Geometry check sheet. Reference: drawing and pictorial views, mm from the part's lowest x, y, z. A direction names the side the tool comes from. Round coordinates to 2 decimals unless told otherwise and drop trailing zeros. Write each loop counter-clockwise with the first axis right and the second up, starting at its lowest first coordinate (ties: lowest second). Pieces come first, ordered by that corner, then holes. Notation, with made-up numbers: M 83,-23.75 L 133,-23.75 A23 cw 133,-8.75 Z; hole C 57.5,89.25 d1. An arc over 180 degrees is marked long. Put each result on its own line as item: value. Start each with the question number.
(1) Tool access check on the marked faces 1, 2 and 3. Record the directions out of +Z, -Z, +X, -X, +Y, -Y that give a thin tool (end or side, any length) a straight path to the whole face; none if there is none.
(2) Section check A-A on z = 38.1. Record the cut outline in (x, y) (3 decimals).
(3) Section check B-B on x = 39. Record the cut outline in (y, z).
(4) Gauge pin test, flat ends, axial feed: pin 1 (6 mm diameter, centred on x = 83, z = 34, fed in from -Y); pin 2 (12 mm diameter, centred on x = 45, z = 63.5, fed in from +Y); pin 3 (12 mm diameter, centred on y = 61, z = 63.5, fed in from +X) (3 decimals). Record the tip position at first contact, or that the pin passes through.
(5) Material ranges on probe 1 along X at (y, z) = (28, 30) (3 decimals); probe 2 along Z at (x, y) = (28.5, 37.5); probe 3 along Y at (x, z) = (55, 60), recorded low to high.
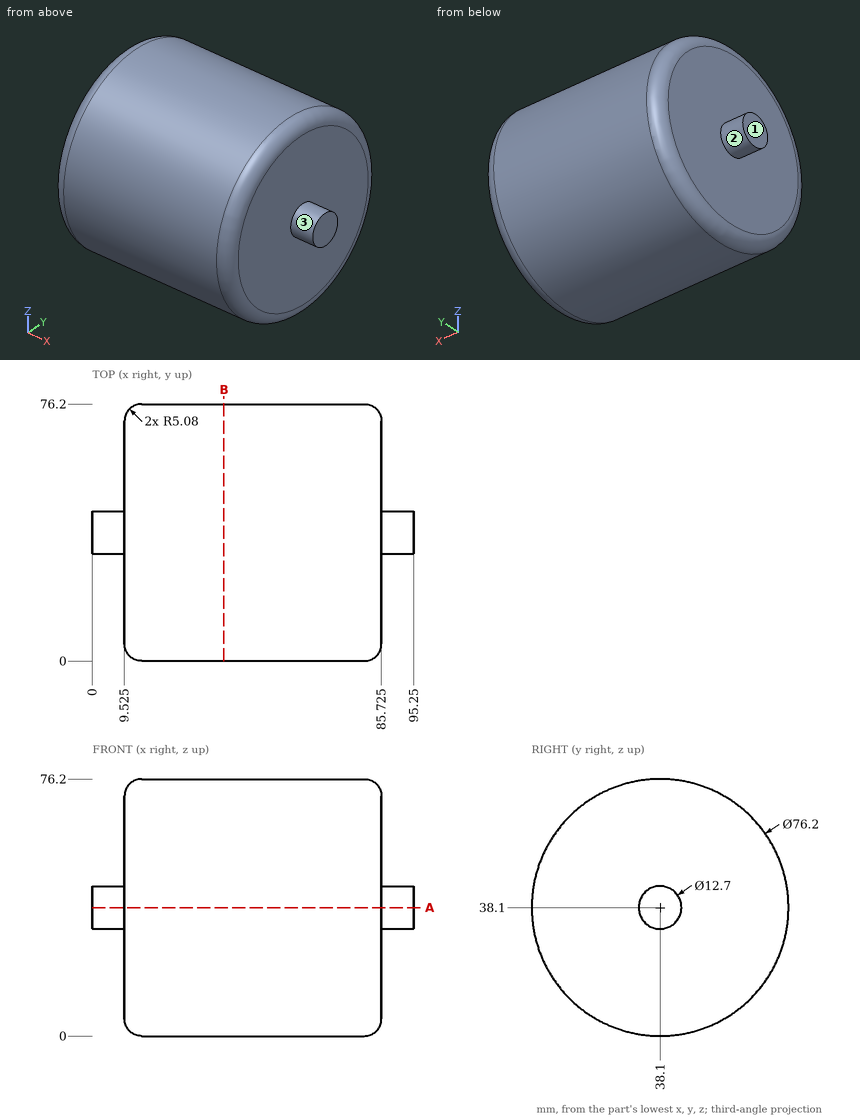
Answers follow:
1. face 1: +Z, -Z, -X, +Y, -Y
1. face 2: -X
1. face 3: +X
2. outline: M 0,31.75 L 9.525,31.75 L 9.525,5.08 A5.08 ccw 14.605,0 L 80.645,0 A5.08 ccw 85.725,5.08 L 85.725,31.75 L 95.25,31.75 L 95.25,44.45 L 85.725,44.45 L 85.725,71.12 A5.08 ccw 80.645,76.2 L 14.605,76.2 A5.08 ccw 9.525,71.12 L 9.525,44.45 L 0,44.45 Z
3. outline: C 38.1,38.1 d76.2
4. pin 1: stops at y = 0.06
4. pin 2: stops at y = 70.89
4. pin 3: stops at x = 85.725
5. probe 1: x = 9.525 to 85.725
5. probe 2: z = 0 to 76.2
5. probe 3: y = 6.92 to 69.28
